from build123d import *

# Parameters (mm, degrees)
PAD_DEPTH    = 895
SKETCH001_R  = 2.5
POCKET_DEPTH = 5


with BuildPart() as part:
    # Sketch → Pad (new body)
    with BuildSketch(Plane.XY):
        with BuildLine():
            Line((10.647392, 10.903953), (12.647392, 10.903953))
            Line((12.647392, 10.903953), (12.647392, -14.096047))
            ThreePointArc((7.647392, -19.096047), (11.182926, -17.631581), (12.647392, -14.096047))
            Line((7.647392, -19.096047), (-22.352608, -19.096047))
            Line((-22.352608, -19.096047), (-22.352608, -17.096047))
            Line((-22.352608, -17.096047), (7.647392, -17.096047))
            ThreePointArc((7.647392, -17.096047), (9.768712, -16.217368), (10.647392, -14.096047))
            Line((10.647392, -14.096047), (10.647392, 10.903953))
        make_face()
    extrude(amount=PAD_DEPTH)

    # Sketch001 → Pocket (cut)
    with BuildSketch(Plane(origin=(10.647392, 0, 0), x_dir=(0, -1, 0), z_dir=(-1, 0, 0))):
        with Locations((1.596047, 7.5)):
            Circle(SKETCH001_R)
        with Locations((1.596047, 456)):
            Circle(SKETCH001_R)
        with Locations((1.596047, 887.5)):
            Circle(SKETCH001_R)
    extrude(amount=-POCKET_DEPTH, mode=Mode.SUBTRACT)


solid = part.part
The listing builds one solid part. Answer for the finished solid, in the listing's coordinates (mm). A direction names the side the tool comes from. Coordinates: 2 decimals unless noted, no trailing zeros. Loops run counter-clockwise (first coordinate to the right, second up) from the corner with the lowest first, then second, coordinate; pieces in that order, holes last. Notation, with made-up numbers: M 10.5,32.25 L 47.5,32.25 A12 ccw 47.5,50.25 Z; hole C 2,-37.5 d7. An arc over 180 degrees is marked long. Answer in a Markdown table with one row per item.
1) Find section B-B (x = -4). Determine the outline of the cut face in (y, z), then the cut area to 3 significant figures.
Answers below:
| item | result |
|---|---|
| outline | M -19.1,0 L -17.1,0 L -17.1,895 L -19.1,895 Z |
| area | 1,790 mm^2 |
2) Which of the six approach directions +Z, -Z, +X, -X, +Y, -Y give full straight-line access (tool end or side, diameter ignored) to faces 1 (the flat face through (10.647, -2, 441)), 2 (the flat face through (3, -17.4, 0))?
Answers below:
| item | result |
|---|---|
| face 1 | +Z, -Z, -X, +Y |
| face 2 | -Z, +X, -X, +Y, -Y |
3) Given pin 1 (5 mm diameter, centred on x = -12, z = 518, fed in from +Y); pin 2 (2 mm diameter, centred on x = -14, y = -14.5, fed in from -Z); pin 3 (12.5 mm diameter, centred on y = -5, z = 659, fed in from -X), each flat-ended and moving along its own axis, determine where each tip first touches the part or whether it passes through.
Answers below:
| item | result |
|---|---|
| pin 1 | y = -17.1 |
| pin 2 | through |
| pin 3 | x = 10.65 |
4) Find section A-A (z = 539). Determine the outline of the cut face in (x, y).
Answers below:
| item | result |
|---|---|
| outline | M -22.35,-19.1 L 7.65,-19.1 A5 ccw 12.65,-14.1 L 12.65,10.9 L 10.65,10.9 L 10.65,-14.1 A3 cw 7.65,-17.1 L -22.35,-17.1 Z |
5) Find the intervals of material crossed by probe 1 along X at (y, z) = (5, 219); probe 2 along Y at (x, z) = (-9, 285); probe 3 along X at (y, z) = (-15, 800.5) (3 decimals), in increasing order.
Answers below:
| item | result |
|---|---|
| probe 1 | 10.65 to 12.65 |
| probe 2 | -19.1 to -17.1 |
| probe 3 | 10.508 to 12.565 |
